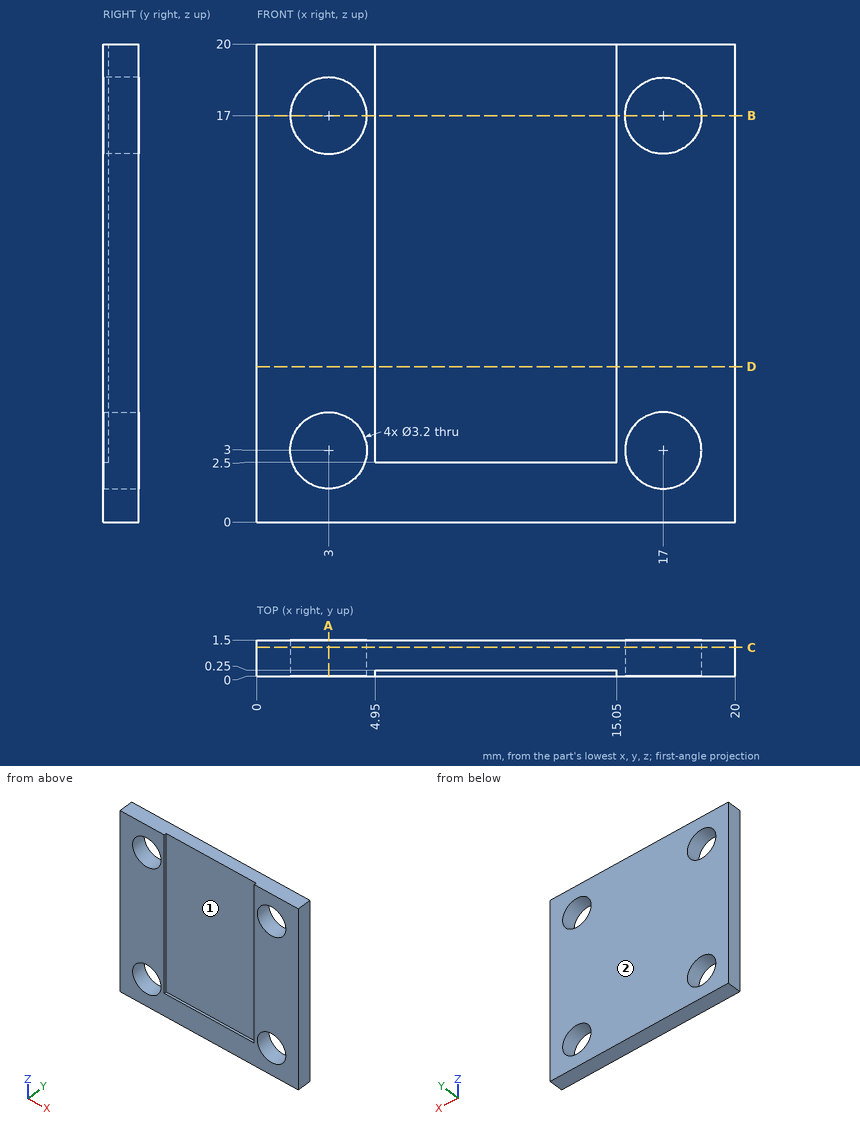
The drawing under review shows one solid part. Ordinate dimensions are in mm from its lowest x, y, z. Give positions to 0.01 mm unless a question says otherwise; leave off trailing zeros. Loops run counter-clockwise (first coordinate to the right, second up) from the corner with the lowest first, then second, coordinate; pieces in that order, holes last. Notation, with made-up numbers: M 8,78 L 40,78 A17 cw 40,92 Z; hole C -5,89.5 d5. An arc over 180 degrees is marked long. Return JSON: item names as keys, results as strings. Group by question number.
Item 1: We need section C-C (y = 1.2). Give the boundary of the cut face in (x, z).
Item 2: We need section A-A (x = 3). Give the boundary of the cut face in (y, z), and give its area (3 significant figures).
Item 3: For probe 1 along X at (y, z) = (0.9, 3); probe 2 along Z at (x, y) = (2.5, 1.25), list the stretches that pass through material, from the lowest coordinate up.
Item 4: Mouldability with a two-part tool opening along Y and no side actions: class the marked faces 1 and 2 as released by +Y, released by -Y, zero draft, split by the parting line, or undercut.
Item 5: We need section B-B (z = 17). Give the boundary of the cut face in (x, y).
Item 6: Insertion check: pin 1 Ø3 at (x, z) = (9.5, 9.5) entering from -Y; pin 2 Ø1.9 at (x, z) = (17, 3) entering from +Y. Each pin has a flat end and moves straight along its axis. Give the tip position at first contact, or say it passes through.
Item 7: We need section D-D (z = 6.5). Give the boundary of the cut face in (x, y).
Output:
{
 "1": {"outline": "M 0,0 L 20,0 L 20,20 L 0,20 Z; hole C 3,3 d3.2; hole C 3,17 d3.2; hole C 17,3 d3.2; hole C 17,17 d3.2"},
 "2": {"outline": "M 0,0 L 1.5,0 L 1.5,1.4 L 0,1.4 Z; M 0,4.6 L 1.5,4.6 L 1.5,15.4 L 0,15.4 Z; M 0,18.6 L 1.5,18.6 L 1.5,20 L 0,20 Z", "area": "20.4 mm^2"},
 "3": {"probe 1": "x = 0 to 1.4, 4.6 to 15.4, 18.6 to 20", "probe 2": "z = 0 to 1.48, 4.52 to 15.48, 18.52 to 20"},
 "4": {"face 1": "released by -Y", "face 2": "released by +Y"},
 "5": {"outline": "M 0,0 L 1.4,0 L 1.4,1.5 L 0,1.5 Z; M 4.6,0 L 4.95,0 L 4.95,0.25 L 15.05,0.25 L 15.05,0 L 15.4,0 L 15.4,1.5 L 4.6,1.5 Z; M 18.6,0 L 20,0 L 20,1.5 L 18.6,1.5 Z"},
 "6": {"pin 1": "stops at y = 0.25", "pin 2": "passes through"},
 "7": {"outline": "M 0,0 L 4.95,0 L 4.95,0.25 L 15.05,0.25 L 15.05,0 L 20,0 L 20,1.5 L 0,1.5 Z"}
}
